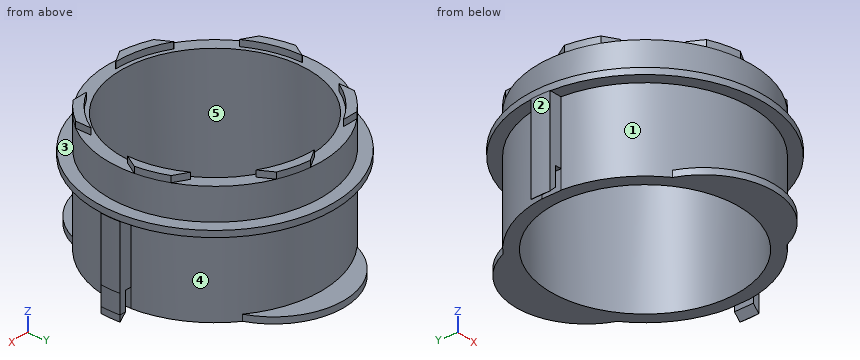
from build123d import *
from OCP.BRepAlgoAPI import BRepAlgoAPI_Cut
from OCP.TopTools import TopTools_ListOfShape
from build123d.topology import SkipClean

# Parameters (mm, degrees)
SKETCH1_R           = 17
BOSS_EXTRUDE1_DEPTH = 19
BOSS_EXTRUDE3_DEPTH = 1
CIRPATTERN1_COUNT   = 6
BOSS_EXTRUDE4_START = -13
BOSS_EXTRUDE4_DEPTH = 14
CUT_EXTRUDE3_START  = -4
CUT_EXTRUDE3_DEPTH  = 4
CHAMFER1_SIZE       = 1
MIRROR1_START       = -1
MIRROR1_DEPTH       = 4
MIRROR1_START_2     = 3
MIRROR1_2_DEPTH     = 10
MIRROR1_3_DEPTH     = 3
MIRROR1_4_DEPTH     = 10
MIRROR1_5_DEPTH     = 1
MIRROR1_START_3     = 11.973929824
MIRROR1_6_OUTLINE_W = 2.659800733000001
MIRROR1_6_OUTLINE_H = 4.5
MIRROR1_6_DEPTH     = 2.142099975
SKETCH7_R           = 18.903661893109657
BOSS_EXTRUDE5_DEPTH = 1
BOSS_EXTRUDE7_DEPTH = 1
SKETCH2_R           = 15.000000000000002
CUT_EXTRUDE5_DEPTH  = 39


with BuildPart() as part:
    # Sketch1 → Boss-Extrude1 (new body)
    with BuildSketch(Plane.XY):
        Circle(SKETCH1_R)
    extrude(amount=BOSS_EXTRUDE1_DEPTH)

    # Sketch4 → Boss-Extrude3 (add)
    with SkipClean():  # the faces are left unmerged after this step: merging them gives an invalid solid
        with BuildSketch(Plane.XY.offset(19)):
            with BuildLine():
                Line((-10.170952539104004, 13.621737203723095), (-7.713345385435483, 13.621737203723095))
                Line((-7.713345385435483, 13.621737203723095), (-7.736883673253982, 13.598198915904591))
                ThreePointArc((-7.736883673253982, 13.598198915904591), (-11.062784069346495, 11.062784069346478), (-13.598198915904605, 7.736883673253956))
                Line((-13.598198915904605, 7.736883673253956), (-13.621737203723118, 7.7133453854354475))
                Line((-13.621737203723118, 7.7133453854354475), (-13.621737203723118, 10.17095253910397))
                ThreePointArc((-13.621737203723118, 10.17095253910397), (-12.020815280171325, 12.020815280171297), (-10.170952539104004, 13.621737203723095))
            make_face()
        boss_extrude3 = extrude(amount=BOSS_EXTRUDE3_DEPTH)

    # CirPattern1: Boss-Extrude3 ×6 about axis
    with SkipClean():  # the faces are left unmerged after this step: merging them gives an invalid solid
        cirpattern1_axis = Axis((-2.8e-16, 1e-17, 0), (0, 0, 1))
        for i in range(1, CIRPATTERN1_COUNT):
            add(boss_extrude3.rotate(cirpattern1_axis, i * 360 / CIRPATTERN1_COUNT))

    # Sketch5 → Boss-Extrude4 (add)
    with SkipClean():  # the faces are left unmerged after this step: merging them gives an invalid solid
        with BuildSketch(Plane(origin=(0, 0, 0), x_dir=(-1, 0, 0), z_dir=(0, 0, -1)).offset(BOSS_EXTRUDE4_START)):
            with BuildLine():
                Line((16.903661893109657, 1.5), (18.903661893109657, 1.5))
                ThreePointArc((18.903661893109657, 1.5), (18.963080787915402, 0), (18.903661893109657, -1.5))
                Line((18.903661893109657, -1.5), (16.903661893109657, -1.5))
                Line((16.903661893109657, -1.5), (16.903661893109657, 1.5))
            make_face()
        extrude(amount=BOSS_EXTRUDE4_DEPTH)


with BuildPart() as cut_extrude3_tool:
    # Cut-Extrude3: read off the stored shape, not the designer's step
    # Cut-Extrude3 outline → Cut-Extrude3 (new body)
    with BuildSketch(Plane(origin=(0, 0, -1), x_dir=(-1, 0, 0), z_dir=(0, 0, -1)).offset(CUT_EXTRUDE3_START)):
        Polygon((17.903661893, 1.5), (16.903661893, 1.500007564), (16.903661893, -1.5), (17.903661893, -1.5), align=None)
    extrude(amount=CUT_EXTRUDE3_DEPTH)


with BuildPart() as part_1:
    add(part.part)

    # Cut-Extrude3: cut by cut_extrude3_tool, with a tolerance
    cut_extrude3_stock = TopTools_ListOfShape()
    cut_extrude3_stock.Append(part_1.part.wrapped)
    cut_extrude3_tools = TopTools_ListOfShape()
    cut_extrude3_tools.Append(cut_extrude3_tool.part.wrapped)
    cut_extrude3_cut = BRepAlgoAPI_Cut()
    cut_extrude3_cut.SetArguments(cut_extrude3_stock)
    cut_extrude3_cut.SetTools(cut_extrude3_tools)
    cut_extrude3_cut.SetFuzzyValue(0.00001)
    cut_extrude3_cut.Build()
    add(Compound.cast(cut_extrude3_cut.Shape()).solids(), mode=Mode.REPLACE)

    # Chamfer1
    chamfer1_edges = [part_1.edges().sort_by_distance(p)[0] for p in [
        (-17.903661893, 0, -1),
    ]]
    chamfer(chamfer1_edges, length=CHAMFER1_SIZE)


with BuildPart() as mirror1_tool:
    # Mirror1: read off the stored shape, not the designer's step
    # Mirror1 outline → Mirror1 (new body)
    with BuildSketch(Plane.XY.offset(MIRROR1_START)):
        Polygon((16.903661893, -1.5), (17.903661893, -1.5), (17.903661893, 1.5), (16.933693552, 1.5), (16.903661893, 1.500015127), align=None)
    extrude(amount=MIRROR1_DEPTH)


with BuildPart() as part_2:
    add(part_1.part)

    # Mirror1: cut by mirror1_tool, with a tolerance
    mirror1_stock = TopTools_ListOfShape()
    mirror1_stock.Append(part_2.part.wrapped)
    mirror1_tools = TopTools_ListOfShape()
    mirror1_tools.Append(mirror1_tool.part.wrapped)
    mirror1_cut = BRepAlgoAPI_Cut()
    mirror1_cut.SetArguments(mirror1_stock)
    mirror1_cut.SetTools(mirror1_tools)
    mirror1_cut.SetFuzzyValue(0.00001)
    mirror1_cut.Build()
    add(Compound.cast(mirror1_cut.Shape()).solids(), mode=Mode.REPLACE)


with BuildPart() as mirror1_2_tool:
    # Mirror1 2 outline → Mirror1 2 (new body)
    with SkipClean():  # the faces are left unmerged after this step: merging them gives an invalid solid
        with BuildSketch(Plane.XY.offset(MIRROR1_START_2)):
            Polygon((16.903661893, -1.5), (17.903661893, -1.5), (17.903661893, 1.5), (16.933693552, 1.5), (16.903661893, 1.500015127), align=None)
            with BuildLine():
                Line((17.903661893, 1.5), (17.903661893, -1.5))
                Line((17.903661893, -1.5), (18.903661893, -1.5))
                ThreePointArc((18.903661893, -1.5), (18.963080788, 0), (18.903661893, 1.5))
                Line((18.903661893, 1.5), (17.903661893, 1.5))
            make_face()
        extrude(amount=MIRROR1_2_DEPTH)


with BuildPart() as part_3:
    with SkipClean():  # the faces are left unmerged after this step: merging them gives an invalid solid
        add(part_2.part)


with BuildPart() as part_4:
    # Mirror1 2: joined with mirror1_2_tool
    with SkipClean():  # the faces are left unmerged after this step: merging them gives an invalid solid
        add(part_3.part.fuse(mirror1_2_tool.part, tol=0.00001))


with BuildPart() as mirror1_3_tool:
    # Mirror1 3 outline → Mirror1 3 (new body)
    with SkipClean():  # the faces are left unmerged after this step: merging them gives an invalid solid
        with BuildSketch(Plane.XY):
            with BuildLine():
                Line((17.903661893, 1.5), (17.903661893, -1.5))
                Line((17.903661893, -1.5), (18.903661893, -1.5))
                ThreePointArc((18.903661893, -1.5), (18.963080788, 0), (18.903661893, 1.5))
                Line((18.903661893, 1.5), (17.903661893, 1.5))
            make_face()
        extrude(amount=MIRROR1_3_DEPTH)


with BuildPart() as part_5:
    with SkipClean():  # the faces are left unmerged after this step: merging them gives an invalid solid
        add(part_4.part)


with BuildPart() as part_6:
    # Mirror1 3: joined with mirror1_3_tool
    with SkipClean():  # the faces are left unmerged after this step: merging them gives an invalid solid
        add(part_5.part.fuse(mirror1_3_tool.part, tol=0.00001))


with BuildPart() as mirror1_4_tool:
    # Mirror1 4 outline → Mirror1 4 (new body)
    with SkipClean():  # the faces are left unmerged after this step: merging them gives an invalid solid
        with BuildSketch(Plane.XY.offset(MIRROR1_START_2)):
            with BuildLine():
                ThreePointArc((16.933693952, 1.500003049), (17, 1.53e-06), (16.933694222, -1.5))
                Line((16.933694222, -1.5), (18.903661893, -1.5))
                ThreePointArc((18.903661893, -1.5), (18.963080788, 0), (18.903661893, 1.5))
                Line((18.903661893, 1.5), (16.933693952, 1.500003049))
            make_face()
        extrude(amount=MIRROR1_4_DEPTH)


with BuildPart() as part_7:
    with SkipClean():  # the faces are left unmerged after this step: merging them gives an invalid solid
        add(part_6.part)


with BuildPart() as part_8:
    # Mirror1 4: joined with mirror1_4_tool
    with SkipClean():  # the faces are left unmerged after this step: merging them gives an invalid solid
        add(part_7.part.fuse(mirror1_4_tool.part, tol=0.00001))


with BuildPart() as mirror1_5_tool:
    # Mirror1 5 outline → Mirror1 5 (new body)
    with SkipClean():  # the faces are left unmerged after this step: merging them gives an invalid solid
        with BuildSketch(Plane.XY.offset(MIRROR1_START)):
            with BuildLine():
                ThreePointArc((16.933693952, 1.500003049), (17, 1.53e-06), (16.933694222, -1.5))
                Line((16.933694222, -1.5), (18.903661893, -1.5))
                ThreePointArc((18.903661893, -1.5), (18.963080788, 0), (18.903661893, 1.5))
                Line((18.903661893, 1.5), (16.933693952, 1.500003049))
            make_face()
        extrude(amount=MIRROR1_5_DEPTH)


with BuildPart() as part_9:
    with SkipClean():  # the faces are left unmerged after this step: merging them gives an invalid solid
        add(part_8.part)


with BuildPart() as part_10:
    # Mirror1 5: joined with mirror1_5_tool
    with SkipClean():  # the faces are left unmerged after this step: merging them gives an invalid solid
        add(part_9.part.fuse(mirror1_5_tool.part, tol=0.00001))


with BuildPart() as mirror1_6_tool:
    # Mirror1 6 outline → Mirror1 6 (new body)
    with BuildSketch(Plane(origin=(0, 0, 0), x_dir=(0.707106781186545, 0, 0.70710678118655), z_dir=(0.70710678118655, 0, -0.707106781186545)).offset(MIRROR1_START_3)):
        with Locations((11.3299003665, 0.75)):
            Rectangle(MIRROR1_6_OUTLINE_W, MIRROR1_6_OUTLINE_H)
    extrude(amount=MIRROR1_6_DEPTH)


with BuildPart() as part_11:
    add(part_10.part)

    # Mirror1 6: cut by mirror1_6_tool, with a tolerance
    mirror1_6_stock = TopTools_ListOfShape()
    mirror1_6_stock.Append(part_11.part.wrapped)
    mirror1_6_tools = TopTools_ListOfShape()
    mirror1_6_tools.Append(mirror1_6_tool.part.wrapped)
    mirror1_6_cut = BRepAlgoAPI_Cut()
    mirror1_6_cut.SetArguments(mirror1_6_stock)
    mirror1_6_cut.SetTools(mirror1_6_tools)
    mirror1_6_cut.SetFuzzyValue(0.00001)
    mirror1_6_cut.Build()
    add(Compound.cast(mirror1_6_cut.Shape()).solids(), mode=Mode.REPLACE)

    # Sketch7 → Boss-Extrude5 (add)
    with SkipClean():  # the faces are left unmerged after this step: merging them gives an invalid solid
        with BuildSketch(Plane.XY.offset(13)):
            with Locations(Location((0, 0, 0), (0, 0, 175.448812236))):
                Circle(SKETCH7_R)
        extrude(amount=BOSS_EXTRUDE5_DEPTH)

    # Sketch11 → Boss-Extrude7 (add)
    with SkipClean():  # the faces are left unmerged after this step: merging them gives an invalid solid
        with BuildSketch(Plane(origin=(0, 0, 0), x_dir=(-1, 0, 0), z_dir=(0, 0, -1))):
            with BuildLine():
                Line((11.160404315577848, 9.320876818848085), (11.160404315577848, -9.320876818848085))
                ThreePointArc((11.160404315577848, -9.320876818848085), (-2.05e-15, -20.481281134425934), (-11.160404315577848, -9.320876818848085))
                Line((-11.160404315577848, -9.320876818848085), (-11.160404315577848, 9.320876818848085))
                ThreePointArc((-11.160404315577848, 9.320876818848085), (6.8e-16, 20.481281134425934), (11.160404315577848, 9.320876818848085))
            make_face()
        extrude(amount=-BOSS_EXTRUDE7_DEPTH)

    # Sketch2 → Cut-Extrude5 (cut)
    with SkipClean():  # the faces are left unmerged after this step: merging them gives an invalid solid
        with BuildSketch(Plane(origin=(0, 0, 0), x_dir=(-1, 0, 0), z_dir=(0, 0, -1))):
            Circle(SKETCH2_R)
        extrude(amount=-CUT_EXTRUDE5_DEPTH, mode=Mode.SUBTRACT)


solid = part_11.part
Source: CAD feature listing. Evaluate the final solid. Frame: model axes, mm. Face numbers are marked on the shaded views. A direction names the side the tool comes from. Give positions to 0.01 mm unless a question says otherwise; leave off trailing zeros. Write each loop counter-clockwise with the first axis right and the second up, starting at its lowest first coordinate (ties: lowest second). Pieces come first, ordered by that corner, then holes. Notation, with made-up numbers: M -17.5,88 L -4.5,88 A13 cw -4.5,108 Z; hole C 42.25,-35 d4. An arc over 180 degrees is marked long. Return JSON: item names as keys, results as strings. Group by question number.
1) Cut plane A-A, the plane y = -13. Output: boundary loops of the cut face in (x, z).
2) Material intervals for line 1 along X through (y, z) = (0.5, 12.5); line 2 along Y through (x, z) = (0, 13.75); line 3 along Z through (x, y) = (3.5, 16), sorted ascending. Write a range as [from, to].
3) Cut plane B-B, the plane x = 1. Output: boundary loops of the cut face in (y, z).
4) Cut plane D-D, the plane x = -8.5. Output: boundary loops of the cut face in (y, z), plus the area to 3 significant figures.
5) Pull-direction query (Z, two-part tool) for the marked faces 1, 2 and 3; classes: pulls with the +Z half, pulls with the -Z half, needs draft (parallel to the pull), parting line crosses it, or undercut.
6) Pin query (flat end, axial travel): P1, Ø2, axis at x = 12, z = 10.5, coming from the -Y side; P2, Ø1, axis at x = -1.5, z = 8, coming from the +Y side; P3, Ø3, axis at x = -14, y = -12, coming from the +Z side. Return the tip coordinate at first contact, or that it passes through.
7) Set-up query: the marked faces 4 and 5. Return all of +Z, -Z, +X, -X, +Y, -Y with unobstructed straight access to the full face (end or side cutting, diameter ignored); none if empty.
Recorded:
{
 "1": {"outline": "M -13.72,13 L -10.95,13 L -10.95,0 L -7.48,0 L -7.48,19 L -10.95,19 L -10.95,14 L -13.72,14 Z; M 7.48,0 L 10.95,0 L 10.95,13 L 13.72,13 L 13.72,14 L 10.95,14 L 10.95,20 L 8.7,20 L 8.7,19 L 7.48,19 Z"},
 "2": {"line 1": "x = [-18.96, -14.99], [14.99, 18.96]", "line 2": "y = [-18.9, -15], [15, 18.9]", "line 3": "z = [0, 20]"},
 "3": {"outline": "M -20.44,0 L -14.97,0 L -14.97,19 L -16.97,19 L -16.97,14 L -18.88,14 L -18.88,13 L -16.97,13 L -16.97,1 L -20.44,1 Z; M 14.97,0 L 20.44,0 L 20.44,1 L 16.97,1 L 16.97,13 L 18.88,13 L 18.88,14 L 16.97,14 L 16.97,19 L 16.31,19 L 16.31,20 L 15.61,20 L 15.61,19 L 14.97,19 Z"},
 "4": {"outline": "M -16.88,13 L -14.72,13 L -14.72,1 L -16.55,1 L -16.55,0 L -12.36,0 L -12.36,19 L -14.72,19 L -14.72,14 L -16.88,14 Z; M 12.36,0 L 16.55,0 L 16.55,1 L 14.72,1 L 14.72,13 L 16.88,13 L 16.88,14 L 14.72,14 L 14.72,19 L 13.62,19 L 13.62,20 L 13.13,20 L 13.13,19 L 12.36,19 Z", "area": "98.3 mm²"},
 "5": {"face 1": "undercut", "face 2": "needs draft", "face 3": "pulls with the +Z half"},
 "6": {"P1": "stops at y = -12.96", "P2": "stops at y = 16.97", "P3": "stops at z = 19"},
 "7": {"face 4": "+Y", "face 5": "+Z, -Z"}
}
